Geometry check sheet. Reference: the model listing, model coordinates, mm. A direction names the side the tool comes from. Round coordinates to 2 decimals unless told otherwise and drop trailing zeros. Order: outer loops, then holes, each group sorted by start corner. A loop starts at its lowest first (then second) coordinate and runs counter-clockwise, first axis right, second up. Notation, with made-up numbers: (55, -21) - (96, -21) arc R15 ccw to (96, -6) - close; hole circle Ø3 at (-32.75, 10.25). An arc over 180 degrees is marked (long way). Use a Markdown table: item, result. Add a question column.
(1) Gauge pin test, flat ends, axial feed: P1, Ø12, axis at y = 23.5, z = -22.5, coming from the -X side; P2, Ø8, axis at y = 31, z = -22.5, coming from the -X side; P3, Ø3, axis at y = 26, z = -18, coming from the -X side; P4, Ø7, axis at x = -21.93, y = 42.19, coming from the +Z side. Record the tip position at first contact, or that the pin passes through.
(2) Thickness scan on line 1 along Z through (x, y) = (-8, 10); line 2 along Z through (x, y) = (-13.25, 32.5); line 3 along X through (y, z) = (31, -39.5). Record the ranges inside material, lowest first. Write a range as [from, to].
(3) Access from +Z, -Z, +X, -X, +Y, -Y to the whole of each face (thin tool, end or side, straight path). Record for faces 3 (the face through (-14.74, 36.69, -21.29)), 4 (the face through (-7.77, 10.88, -44.03)), 5 (the face through (-8.552, 17.673, -20.706)).
(4) Mould release check, pull along Z, two halves, no side actions. Record for faces 1 (the face through (-14, 26, -42)), 2 (the face through (-13.074, 6.559, 2.028)): released by +Z, released by -Z, zero draft, split by the parting line, or undercut.
(5) Section check A-A on y = 44. Record the boundary of the cut face in (x, z), then the cut area to 3 significant figures.
(6) Section check D-D on x = -20.25. Record the boundary of the cut face in (y, z).
(7) Section check C-C on z = -36. Record the boundary of the cut face in (x, y), then the cut area to 3 significant figures.
(8) Section check B-B on y = 16. Record the boundary of the cut face in (x, z).
```python
from build123d import *

# Parameters (mm, degrees)
BOSS_EXTRUDE1_DEPTH          = 5
SKETCH6_W                    = 42
SKETCH6_H                    = 20
BOSS_EXTRUDE2_DEPTH          = 3
BOSS_EXTRUDE3_DEPTH          = 4
SKETCH14_W                   = 3
SKETCH14_H                   = 42
BOSS_EXTRUDE4_DEPTH          = 3
SKETCH15_W                   = 3
SKETCH15_H                   = 42
CUT_EXTRUDE1_DEPTH           = 3
BOSS_EXTRUDE5_DEPTH          = 4
F_2_0_2_DIAMETER_HOLE1_D     = 2
F_2_0_2_DIAMETER_HOLE1_DEPTH = 13.574856707
F_4_0_4_DIAMETER_HOLE1_D     = 4
F_4_0_4_DIAMETER_HOLE1_DEPTH = 13.574856707
HOLE1_D                      = 5.275
HOLE1_DEPTH                  = 4
HOLE2_D                      = 5.275
HOLE2_DEPTH                  = 4
F_3_0_3_DIAMETER_HOLE1_D     = 3
F_3_0_3_DIAMETER_HOLE1_DEPTH = 26.254229339
FILLET1_R                    = 3


with BuildPart() as part:
    # Sketch1 → Boss-Extrude1 (new body)
    with BuildSketch(Plane(origin=(-8.342407099, 25.628804584, 0), x_dir=(0.950891688, 0.309523823, 0), z_dir=(0.309523823, -0.950891688, 0))):
        with BuildLine():
            Line((-4.14030738, -30.713017444), (-4.14030738, -23.589232886))
            add(Edge.make_bspline(
                [(-4.14030738, -23.589232886), (-4.220798256, -24.279493403), (-4.802543831, -24.911473889), (-5.885544107, -25.485174345)],
                knots=[0, 0, 0, 0, 1, 1, 1, 1], degree=3))
            ThreePointArc((-5.885544107, -25.485174345), (-7.885544107, -27.485174345), (-5.885544107, -29.485174345))
            add(Edge.make_bspline(
                [(-5.885544107, -29.485174345), (-4.984417634, -29.728649028), (-4.402672059, -30.137930061), (-4.14030738, -30.713017444)],
                knots=[0, 0, 0, 0, 1, 1, 1, 1], degree=3))
        make_face()
    extrude(amount=-BOSS_EXTRUDE1_DEPTH)

    # Sketch6 → Boss-Extrude2 (add)
    with BuildSketch(Plane(origin=(-3.936983875, -1.281523768, 0), x_dir=(0, 0, 1), z_dir=(-0.950891688, -0.309523823, 0))):
        with Locations((-21, 29.452391)):
            Rectangle(SKETCH6_W, SKETCH6_H)
    extrude(amount=-BOSS_EXTRUDE2_DEPTH)

    # Sketch8 → Boss-Extrude3 (add)
    with BuildSketch(Plane.XY):
        with BuildLine():
            Line((-17.397624454, 40.071064625), (-17.077010229, 39.086101986))
            ThreePointArc((-17.077010229, 39.086101986), (-15.584881864, 37.340928389), (-13.295763695, 37.161998389))
            Line((-13.295763695, 37.161998389), (-7.105287237, 18.144164622))
            ThreePointArc((-7.105287237, 18.144164622), (-8.850460834, 16.652036257), (-9.029390833, 14.362918088))
            Line((-9.029390833, 14.362918088), (-7.842362425, 10.716234493))
            ThreePointArc((-7.842362425, 10.716234493), (-11.874437039, 1.653788416), (-10.256851829, 11.439950722))
            Line((-10.256851829, 11.439950722), (-18.956793202, 38.167140452))
            ThreePointArc((-18.956793202, 38.167140452), (-25.795005306, 45.357497095), (-17.397624454, 40.071064625))
        make_face()
    extrude(amount=BOSS_EXTRUDE3_DEPTH)

    # Sketch14 → Boss-Extrude4 (add)
    with BuildSketch(Plane(origin=(-6.020978427, 18.497116921, 0), x_dir=(-0.950891688, -0.309523823, 0), z_dir=(0.309523823, -0.950891688, 0))):
        with Locations((2.64030738, 21)):
            Rectangle(SKETCH14_W, SKETCH14_H)
    extrude(amount=BOSS_EXTRUDE4_DEPTH)

    # Sketch15 → Cut-Extrude1 (cut)
    with BuildSketch(Plane(origin=(-5.092406958, 15.644441856, 0), x_dir=(0.950891688, 0.309523823, 0), z_dir=(0.309523823, -0.950891688, 0))):
        with Locations((-2.64030738, -21)):
            Rectangle(SKETCH15_W, SKETCH15_H)
    extrude(amount=-CUT_EXTRUDE1_DEPTH, mode=Mode.SUBTRACT)

    # Sketch22 → Boss-Extrude5 (add)
    with BuildSketch(Plane(origin=(0, 0, -42), x_dir=(-1, 0, 0), z_dir=(0, 0, -1))):
        with BuildLine():
            Line((18.956793202, 38.167140452), (10.256851829, 11.439950722))
            ThreePointArc((10.256851829, 11.439950722), (11.874437039, 1.653788416), (7.842362425, 10.716234493))
            Line((7.842362425, 10.716234493), (9.029390833, 14.362918088))
            ThreePointArc((9.029390833, 14.362918088), (8.850460834, 16.652036257), (7.105287237, 18.144164622))
            Line((7.105287237, 18.144164622), (13.295763695, 37.161998389))
            ThreePointArc((13.295763695, 37.161998389), (15.584881864, 37.340928389), (17.077010229, 39.086101986))
            Line((17.077010229, 39.086101986), (17.397624454, 40.071064625))
            ThreePointArc((17.397624454, 40.071064625), (25.795005306, 45.357497095), (18.956793202, 38.167140452))
        make_face()
    extrude(amount=BOSS_EXTRUDE5_DEPTH)

    # Ø2.0 (2) Diameter Hole1
    with Locations(Plane(origin=(-3.936983875, -1.281523768, 0), x_dir=(0, 0, 1), z_dir=(-0.950891688, -0.309523823, 0))):
        with Locations((-21, 29.452391)):
            Hole(F_2_0_2_DIAMETER_HOLE1_D / 2, depth=F_2_0_2_DIAMETER_HOLE1_DEPTH)

    # Ø4.0 (4) Diameter Hole1
    with Locations(Plane(origin=(-3.936983875, -1.281523768, 0), x_dir=(0, 0, 1), z_dir=(-0.950891688, -0.309523823, 0))):
        with Locations((-5, 24.452391), (-37, 24.452391), (-37, 34.452391), (-5, 34.452391)):
            Hole(F_4_0_4_DIAMETER_HOLE1_D / 2, depth=F_4_0_4_DIAMETER_HOLE1_DEPTH)

    # Hole1
    with Locations(Plane(origin=(0, 0, -46), x_dir=(-1, 0, 0), z_dir=(0, 0, -1))):
        with Locations((10.438845238, 6.44326398), (21.926625837, 42.189589224)):
            Hole(HOLE1_D / 2, depth=HOLE1_DEPTH)

    # Hole2
    with Locations(Plane(origin=(0, 0, 0), x_dir=(-1, 0, 0), z_dir=(0, 0, -1))):
        with Locations((10.438845238, 6.44326398), (21.926625837, 42.189589224)):
            Hole(HOLE2_D / 2, depth=HOLE2_DEPTH)

    # Ø3.0 (3) Diameter Hole1
    with Locations(Plane(origin=(-8.342407099, 25.628804584, 0), x_dir=(-0.950891688, -0.309523823, 0), z_dir=(0.309523823, -0.950891688, 0))):
        with Locations((5.885544107, 27.485174345)):
            Hole(F_3_0_3_DIAMETER_HOLE1_D / 2, depth=F_3_0_3_DIAMETER_HOLE1_DEPTH)

    # Fillet1
    fillet1_edges = [part.edges().sort_by_distance(p)[0] for p in [
        (-17.397624454, 40.071064625, 2),
        (-18.956793202, 38.167140452, 2),
        (-10.256851829, 11.439950722, 2),
        (-7.842362425, 10.716234493, 2),
        (-18.956793202, 38.167140452, -44),
        (-17.397624454, 40.071064625, -44),
        (-7.842362425, 10.716234493, -44),
        (-10.256851829, 11.439950722, -44),
    ]]
    fillet(fillet1_edges, radius=FILLET1_R)


solid = part.part
```
Check sheet entries:
| question | item | result |
|---|---|---|
| 1 | P1 | stops at x = -17.18 |
| 1 | P2 | stops at x = -15.96 |
| 1 | P3 | stops at x = -13.31 |
| 1 | P4 | stops at z = 4 |
| 2 | line 1 | z = [-46, -42], [0, 4] |
| 2 | line 2 | z = [-46, -38.92], [-35.08, -6.92], [-3.08, 4] |
| 2 | line 3 | x = [-14.44, -11.29] |
| 3 | face 3 | -X, +Y |
| 3 | face 4 | +Z, -Z, +X |
| 3 | face 5 | +X, -Y |
| 4 | face 1 | undercut |
| 4 | face 2 | zero draft |
| 5 | outline | (-26.59, -46) - (-23.84, -46) - (-23.84, -42) - (-26.59, -42) - close; (-26.59, 0) - (-23.84, 0) - (-23.84, 4) - (-26.59, 4) - close; (-20.01, -46) - (-17.27, -46) - (-17.27, -42) - (-20.01, -42) - close; (-20.01, 0) - (-17.27, 0) - (-17.27, 4) - (-20.01, 4) - close |
| 5 | area | 43.9 mm2 |
| 6 | outline | (37.2, -46) - (40.15, -46) - (40.15, -42) - (37.2, -42) - close; (37.2, 0) - (40.15, 0) - (40.15, 4) - (37.2, 4) - close; (44.23, -46) - (46.9, -46) - (46.9, -42) - (44.23, -42) - close; (44.23, 0) - (46.9, 0) - (46.9, 4) - (44.23, 4) - close |
| 7 | outline | (-16.15, 36.23) - (-15.14, 33.13) - (-12.28, 34.05) - (-13.3, 37.16) - close; (-14.06, 29.83) - (-12.04, 23.62) - (-9.19, 24.55) - (-11.21, 30.76) - close; (-10.97, 20.32) - (-9.96, 17.22) - (-7.11, 18.14) - (-8.12, 21.25) - close |
| 7 | area | 39.2 mm2 |
| 8 | outline | (-11.74, -46) - (-9.09, -46) - (-9.09, -42) - (-11.74, -42) - close; (-11.74, 0) - (-9.09, 0) - (-9.09, 4) - (-11.74, 4) - close |
